Geometry check sheet. Reference: the model listing, model coordinates, mm. A direction names the side the tool comes from. Coordinates: 2 decimals unless noted, no trailing zeros. Write each loop counter-clockwise with the first axis right and the second up, starting at its lowest first coordinate (ties: lowest second). Pieces come first, ordered by that corner, then holes.
Autodesk Inventor part; units mm, degrees
ref_plane "YZ Plane" through (0, 0, 0) normal (1, 0, 0) x (0, 1, 0)
ref_plane "XZ Plane" through (0, 0, 0) normal (0, 1, 0) x (-1, 0, 0)
ref_plane "XY Plane" through (0, 0, 0) normal (0, 0, 1) x (1, 0, 0)
sketch "Sketch1" plane through (0, 0, 0) normal (0, 0, 1) x (1, 0, 0)
  line L0 (-30.5603, 10.2886) -> (29.4397, 10.2886)
  line L1 (29.4397, 10.2886) -> (29.4397, -9.7114)
  line L2 (29.4397, -9.7114) -> (-30.5603, -9.7114)
  line L3 (-30.5603, -9.7114) -> (-30.5603, 10.2886)
  point P0 (0, 0)
  dimension "d0" = 60
  dimension "d1" = 20
extrude "Extrusion1" add sketch "Sketch1" along normal blind 1
sketch "Sketch2" plane through (0, 0, 1) normal (0, 0, 1) x (1, 0, 0)
  line L0 (-30.5603, 10.2886) -> (-30.5603, -9.7114)
  line L1 (-30.5603, 10.2886) -> (29.4397, 10.2886)
  line L2 (29.4397, -9.7114) -> (29.4397, 10.2886)
  point P0 (0, 0)
  point P1 (-13.0603, 0.2886)
  point P2 (11.9397, 0.2886)
  dimension "d4" = 25
  dimension "d5" = 17.5
  dimension "d6" = 10
  dimension "d7" = 10
  dimension "d8" = 17.5
hole "Hole1" at (-13.0603, 0.2886, 1) at (11.9397, 0.2886, 1) direction (0, 0, -1) diameter 3 depth 8 tip angle 118 countersink diameter 6 countersink angle 90
sketch "Sketch3" plane through (0, 0, 1) normal (0, 0, 1) x (1, 0, 0)
  line L0 (-30.5603, 10.2886) -> (-28.5603, 10.2886)
  line L1 (-28.5603, 10.2886) -> (-28.5603, -9.7114)
  line L2 (-28.5603, -9.7114) -> (-30.5603, -9.7114)
  line L3 (-30.5603, -9.7114) -> (-30.5603, 10.2886)
  line L4 (29.4397, 10.2886) -> (27.4397, 10.2886)
  line L5 (27.4397, 10.2886) -> (27.4397, -9.7114)
  line L6 (27.4397, -9.7114) -> (29.4397, -9.7114)
  line L7 (29.4397, -9.7114) -> (29.4397, 10.2886)
  line L8 (-30.5603, -9.7114) -> (29.4397, -9.7114)
  point P0 (0, 0)
  dimension "d16" = 2
  dimension "d17" = 2
extrude "Extrusion2" add sketch "Sketch3" along normal blind 3
chamfer "Chamfer1" distance 2 angle 45 2 edges at (-28.5603, 0.2886, 1) (27.4397, 0.2886, 1)
properties part number "head mount"
1. Sectioned sample at B-B, the plane y = -4.25. Record the boundary of the cut face in (x, z).
Computed values:
outline: (-30.56, 0) - (29.44, 0) - (29.44, 4) - (27.44, 4) - (27.44, 3) - (25.44, 1) - (-26.56, 1) - (-28.56, 3) - (-28.56, 4) - (-30.56, 4) - close
2. Sectioned sample at C-C, the plane y = 1. Give the number of separate pieces and of enclosed holes in the cut face, and give its area (3 significant figures).
Computed values:
separate pieces: 3
enclosed holes: 0
area: 66.4 mm2
3. Thickness scan on line 1 along X through (y, z) = (-6.5, 3.5); line 2 along X through (y, z) = (0.25, 0.45); line 3 along X through (y, z) = (-6.25, 1.35). Record the ranges inside material, lowest first.
Computed values:
line 1: x = -30.56 to -28.56, 27.44 to 29.44
line 2: x = -30.56 to -15.51, -10.61 to 9.49, 14.39 to 29.44
line 3: x = -30.56 to -26.91, 25.79 to 29.44
4. Gauge pin test, flat ends, axial feed: pin 1 Ø8 at (x, y) = (-19, -4.5) entering from -Z; pin 2 Ø10 at (x, y) = (-5, -3) entering from +Z. Record the tip position at first contact, or that the pin passes through.
Computed values:
pin 1: stops at z = 0
pin 2: stops at z = 1
5. Sectioned sample at A-A, the plane z = 2.25. Record the boundary of the cut face in (x, y), and give its area (3 significant figures).
Computed values:
outline: (-30.56, -9.71) - (-27.81, -9.71) - (-27.81, 10.29) - (-30.56, 10.29) - close; (26.69, -9.71) - (29.44, -9.71) - (29.44, 10.29) - (26.69, 10.29) - close
area: 110 mm2
6. Draft check along X on faces 1 (the flat face through (-30.56, 0, 2)), 2 (the flat face through (-1, 0, 0)), 3 (the flat face through (-27.57, 0.43, 2.01)). Enter one of: released by +X, released by -X, zero draft, split by the parting line, or undercut.
Computed values:
face 1: released by -X
face 2: zero draft
face 3: undercut
7. Sectioned sample at D-D, the plane x = -3.5. Record the boundary of the cut face in (y, z).
Computed values:
outline: (-9.71, 0) - (10.29, 0) - (10.29, 1) - (-9.71, 1) - close
8. Access from +Z, -Z, +X, -X, +Y, -Y to the whole of each face (thin tool, end or side, straight path). Record for faces 4 (the flat face through (27.44, 0.4, 3.5)), 5 (the flat face through (29.44, 0, 2)).
Computed values:
face 4: +Z, +Y, -Y
face 5: +Z, -Z, +X, +Y, -Y
